```python
from build123d import *

# Parameters (mm, degrees)
BOSS_EXTRUDE2_DEPTH = 36
BOSS_EXTRUDE3_DEPTH = 66
SKETCH1_7_R         = 25
BOSS_EXTRUDE4_DEPTH = 20
SKETCH1_8_W         = 115
SKETCH1_8_H         = 69
SKETCH1_8_R         = 20
BOSS_EXTRUDE5_DEPTH = 149
SKETCH1_10_W        = 62
SKETCH1_10_H        = 30
BOSS_EXTRUDE6_DEPTH = 20
RIB2_REACH          = 354.463
SKETCH5_WALL_W      = 850.051346756
SKETCH5_WALL_H      = 30


with BuildPart() as part:
    # Sketch1 → Boss-Extrude2 (new body)
    with BuildSketch(Plane(origin=(0, 0, 0), x_dir=(1, 0, 0), z_dir=(0, 1, 0))):
        with BuildLine():
            ThreePointArc((198, 100), (298, 0), (198, -100))
            Line((198, -100), (-198, -100))
            ThreePointArc((-198, -100), (-298, 0), (-198, 100))
            Line((-198, 100), (198, 100))
        make_face()
        with BuildLine():
            ThreePointArc((198, -75), (273, 0), (198, 75))
            Line((198, 75), (-198, 75))
            ThreePointArc((-198, 75), (-273, 0), (-198, -75))
            Line((-198, -75), (198, -75))
        make_face(mode=Mode.SUBTRACT)
    extrude(amount=BOSS_EXTRUDE2_DEPTH)

    # Sketch1<6> → Boss-Extrude3 (add)
    with BuildSketch(Plane(origin=(0, 0, 0), x_dir=(1, 0, 0), z_dir=(0, 1, 0))):
        with BuildLine():
            Line((-198, -75), (198, -75))
            ThreePointArc((198, -75), (273, 0), (198, 75))
            Line((198, 75), (-198, 75))
            ThreePointArc((-198, 75), (-273, 0), (-198, -75))
        make_face()
        with BuildLine():
            Line((-198, 50), (198, 50))
            ThreePointArc((198, 50), (248, 0), (198, -50))
            Line((198, -50), (-198, -50))
            ThreePointArc((-198, -50), (-248, 0), (-198, 50))
        make_face(mode=Mode.SUBTRACT)
    extrude(amount=BOSS_EXTRUDE3_DEPTH)

    # Sketch1<7> → Boss-Extrude4 (add)
    with BuildSketch(Plane(origin=(0, 0, 0), x_dir=(1, 0, 0), z_dir=(0, 1, 0))):
        with BuildLine():
            Line((198, 50), (-198, 50))
            ThreePointArc((-198, 50), (-248, 0), (-198, -50))
            Line((-198, -50), (198, -50))
            ThreePointArc((198, -50), (248, 0), (198, 50))
        make_face()
        with Locations(Location((-198, 0, 0), (0, 0, 270))):
            Circle(SKETCH1_7_R, mode=Mode.SUBTRACT)
        Polygon((57.5, -34.5), (-57.5, -34.5), (-57.5, -15), (-119.5, -15), (-119.5, 15), (-57.5, 15), (-57.5, 34.5), (57.5, 34.5), (57.5, 15), (119.5, 15), (119.5, -15), (57.5, -15), align=None, mode=Mode.SUBTRACT)
        with Locations(Location((198, 0, 0), (0, 0, 270))):
            Circle(SKETCH1_7_R, mode=Mode.SUBTRACT)
    extrude(amount=BOSS_EXTRUDE4_DEPTH)

    # Sketch1<8> → Boss-Extrude5 (add)
    with BuildSketch(Plane(origin=(0, 0, 0), x_dir=(1, 0, 0), z_dir=(0, 1, 0))):
        Rectangle(SKETCH1_8_W, SKETCH1_8_H)
        with Locations(Location((0, 0, 0), (0, 0, 270))):
            Circle(SKETCH1_8_R, mode=Mode.SUBTRACT)
    extrude(amount=BOSS_EXTRUDE5_DEPTH)

    # Sketch1<10> → Boss-Extrude6 (add)
    with BuildSketch(Plane(origin=(0, 0, 0), x_dir=(1, 0, 0), z_dir=(0, 1, 0))):
        with Locations((-88.5, 0)):
            Rectangle(SKETCH1_10_W, SKETCH1_10_H)
        with Locations((88.5, 0)):
            Rectangle(SKETCH1_10_W, SKETCH1_10_H)
    extrude(amount=BOSS_EXTRUDE6_DEPTH)

    # Sketch5 wall → Rib2 (add, up to next)
    with BuildSketch(Plane(origin=(-88.5, 84.5, 15), x_dir=(0.433185294803, 0.901304887575, 0), z_dir=(0.901304887575, -0.433185294803, 0)), mode=Mode.PRIVATE) as rib2_sk1:
        with Locations((0, -15)):
            Rectangle(SKETCH5_WALL_W, SKETCH5_WALL_H)
    rib2_tool1 = extrude(rib2_sk1.sketch, amount=RIB2_REACH, mode=Mode.PRIVATE) - part.part
    rib2 = rib2_tool1.solids().sort_by_distance((-88.5, 84.5, 15))[0]
    add(rib2)

    # Mirror1: Rib2 across plane
    add(rib2.mirror(Plane(origin=(0, 0, 0), x_dir=(0, 0, 1), z_dir=(1, 0, 0))))


solid = part.part
```
Could you check a few things on this model? Use its own coordinates, in mm. A direction names the side the tool comes from. Give positions to 0.01 mm unless a question says otherwise; leave off trailing zeros. Order: outer loops, then holes, each group sorted by start corner. A loop starts at its lowest first (then second) coordinate and runs counter-clockwise, first axis right, second up.
Q1. We'd pull the mould along X, two halves only. Please class faces 1 (the cylindrical face through (-272.98, 50.79, -1.65)), 2 (the flat face through (-57.5, 84, -25)), 3 (the flat face through (-14, 149, -16)): +X half, -X half, draft (parallel to the pull), parting line (faces both ways), or undercut.
Q2. Suppose I cut it at B-B, the plane z = 0. Write out the boundary of the cut face in (x, y).
Q3. For faces 4 (the cylindrical face through (-173.213, 9.86, -3.255)), 5 (the flat face through (-77, 60, 15)), which set-ups out of +Z, -Z, +X, -X, +Y, -Y let a thin tool reach every point of the face, with its end or its side?
Q4. Suppose I cut it at A-A, the plane y = 60. Write out the boundary of the cut face in (x, z).
Q5. If I drill on line 1 along X through (y, z) = (6, 0); line 2 along Y through (x, z) = (-259.5, 22); line 3 along Y through (x, z) = (231.5, -23), over which ranges is the centre line in solid material (lowest first)?
Q6. Suppose I cut it at D-D, the plane z = -68. Write out the boundary of the cut face in (x, y), and give its area (3 significant figures).
Q7. I'm going to push flat-ended pins straight in: P1, Ø2, axis at x = -79.5, z = 58.5, coming from the +Y side; P2, Ø2, axis at x = -34.5, y = 74, coming from the -Z side; P3, Ø24, axis at x = 94, y = 45, coming from the +Z side; P4, Ø10, axis at y = 92, z = -21, coming from the +X side. Where does each tip first touch, or does it pass through?
Q8. Suppose I cut it at C-C, the plane y = 109. Write out the boundary of the cut face in (x, z).
Solution:
1. face 1: -X half
1. face 2: undercut
1. face 3: draft
2. outline: (-298, 0) - (-223, 0) - (-223, 20) - (-248, 20) - (-248, 66) - (-273, 66) - (-273, 36) - (-298, 36) - close; (-173, 0) - (-20, 0) - (-20, 149) - (-57.5, 149) - (-119.5, 20) - (-173, 20) - close; (20, 0) - (173, 0) - (173, 20) - (119.5, 20) - (57.5, 149) - (20, 149) - close; (223, 0) - (298, 0) - (298, 36) - (273, 36) - (273, 66) - (248, 66) - (248, 20) - (223, 20) - close
3. face 4: +Y, -Y
3. face 5: +Y
4. outline: (-198, -75) - (198, -75) arc R75 ccw to (198, 75) - (-198, 75) arc R75 ccw to start; (-100.28, -15) - (-57.5, -15) - (-57.5, -34.5) - (57.5, -34.5) - (57.5, -15) - (100.28, -15) - (100.28, 15) - (57.5, 15) - (57.5, 34.5) - (-57.5, 34.5) - (-57.5, 15) - (-100.28, 15) - close; hole (-198, -50) - (198, -50) arc R50 ccw to (198, 50) - (-198, 50) arc R50 ccw to start; hole circle Ø40 at (0, 0)
5. line 1: x = -298 to -223, -173 to -20, 20 to 173, 223 to 298
5. line 2: y = 0 to 66
5. line 3: y = 0 to 20
6. outline: (-271.32, 0) - (271.32, 0) - (271.32, 36) - (229.64, 36) - (229.64, 66) - (-229.64, 66) - (-229.64, 36) - (-271.32, 36) - close
6. area: 33,300 mm2
7. P1: stops at y = 66
7. P2: stops at z = -34.5
7. P3: stops at z = 100
7. P4: stops at x = 57.5
8. outline: (-76.72, -15) - (-57.5, -15) - (-57.5, -34.5) - (57.5, -34.5) - (57.5, -15) - (76.72, -15) - (76.72, 15) - (57.5, 15) - (57.5, 34.5) - (-57.5, 34.5) - (-57.5, 15) - (-76.72, 15) - close; hole circle Ø40 at (0, 0)
